```python
from build123d import *

# Parameters (mm, degrees)
SKETCH1_W           = 19.05
SKETCH1_H           = 11.125
BOSS_EXTRUDE1_DEPTH = 3.175
SKETCH2_W           = 3.175
SKETCH2_H           = 1.5875
CUT_EXTRUDE2_DEPTH  = 3.175


with BuildPart() as part:
    # Sketch1 → Boss-Extrude1 (new body)
    with BuildSketch(Plane(origin=(0, 0, 0), x_dir=(1, 0, 0), z_dir=(0, 1, 0))):
        Rectangle(SKETCH1_W, SKETCH1_H)
    extrude(amount=BOSS_EXTRUDE1_DEPTH)

    # Sketch2 → Cut-Extrude2 (cut)
    with BuildSketch(Plane(origin=(0, 3.175, 0), x_dir=(1, 0, 0), z_dir=(0, 1, 0))):
        with Locations((-7.9375, -1.58125)):
            Rectangle(SKETCH2_W, SKETCH2_H)
        with BuildLine():
            ThreePointArc((-6.35, -5.5625), (-8.501887576, -4.726496568), (-9.525, -2.657012854))
            Line((-9.525, -2.657012854), (-9.525, -5.5625))
            Line((-9.525, -5.5625), (-6.35, -5.5625))
        make_face()
        with BuildLine():
            Line((9.525, -5.5625), (9.525, -2.657012854))
            ThreePointArc((9.525, -2.657012854), (8.501887576, -4.726496568), (6.35, -5.5625))
            Line((6.35, -5.5625), (9.525, -5.5625))
        make_face()
        with Locations((7.9375, -1.58125)):
            Rectangle(SKETCH2_W, SKETCH2_H)
    extrude(amount=-CUT_EXTRUDE2_DEPTH, mode=Mode.SUBTRACT)


solid = part.part
```
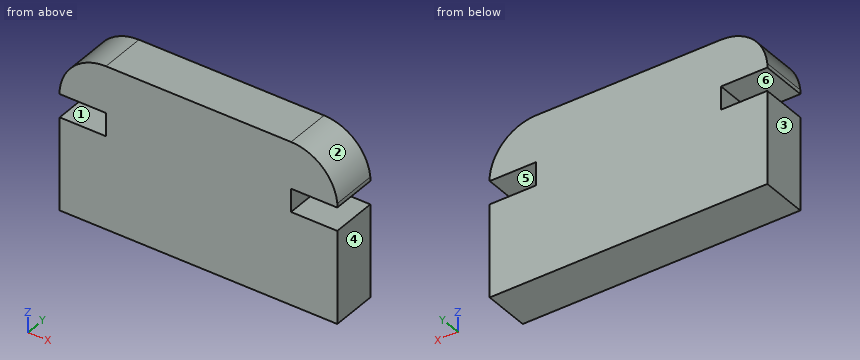
Geometry check sheet. Reference: the model listing, model coordinates, mm. Face numbers are marked on the shaded views. A direction names the side the tool comes from. Coordinates: 2 decimals unless noted, no trailing zeros. Order: outer loops, then holes, each group sorted by start corner. A loop starts at its lowest first (then second) coordinate and runs counter-clockwise, first axis right, second up. Notation, with made-up numbers: (79.25, 1.5) - (137.25, 1.5) arc R24 cw to (137.25, 30.5) - close; hole circle Ø6 at (74, 82.5). An arc over 180 degrees is marked (long way). Use one line per item in the form item = value.
1. Access from +Z, -Z, +X, -X, +Y, -Y to the whole of each face (thin tool, end or side, straight path). Record for the marked faces 4, 5 and 6.
Here are the results:
face_4 = +Z, -Z, +X, +Y, -Y
face_5 = +X, +Y, -Y
face_6 = -X, +Y, -Y
2. Section check D-D (z = 3.5). Record the boundary of the cut face in (x, y) (3 decimals).
Here are the results:
outline = (-9.332, 0) - (9.332, 0) - (9.332, 3.175) - (-9.332, 3.175) - close
3. Scan lines: line 1 (Z direction, x = 6.5, y = 1.1) (1 decimal); line 2 (X direction, y = 1.7, z = 1); line 3 (Z direction, x = 7.75, y = 2.35) (1 decimal). Record each from-to range of solid material in increasing order.
Here are the results:
line_1 = -5.6 to 0.8, 2.4 to 5.6
line_2 = -6.35 to 6.35
line_3 = -5.6 to 0.8, 2.4 to 5.2
4. Gauge pin test, flat ends, axial feed: pin 1 (1.5 mm diameter, centred on x = -3.5, z = -1.5, fed in from -Y); pin 2 (1.3 mm diameter, centred on y = 2, z = 1.5, fed in from -X); pin 3 (0.5 mm diameter, centred on y = 1, z = 2, fed in from +X); pin 4 (1.6 mm diameter, centred on x = -8, y = 2, fed in from +Z). Record the tip position at first contact, or that the pin passes through.
Here are the results:
pin_1 = 0
pin_2 = -6.35
pin_3 = 6.35
pin_4 = 5.45
5. Section check C-C (z = 1.75). Record the boundary of the cut face in (x, y) (3 decimals).
Here are the results:
outline = (-6.35, 0) - (6.35, 0) - (6.35, 3.175) - (-6.35, 3.175) - close
6. Section check A-A (x = -7). Record the boundary of the cut face in (y, z) (1 decimal).
Here are the results:
outline = (0, -5.6) - (3.2, -5.6) - (3.2, 0.8) - (0, 0.8) - close; (0, 2.4) - (3.2, 2.4) - (3.2, 5.5) - (0, 5.5) - close
7. Draft check along Z on the marked faces 1, 2 and 3. Enter one of: pulls with the +Z half, pulls with the -Z half, needs draft (parallel to the pull), parting line crosses it, or undercut.
Here are the results:
face_1 = undercut
face_2 = pulls with the +Z half
face_3 = needs draft
